Could you check a few things on this model? Use its own coordinates, in mm. Round coordinates to 2 decimals unless told otherwise and drop trailing zeros. Order: outer loops, then holes, each group sorted by start corner. A loop starts at its lowest first (then second) coordinate and runs counter-clockwise, first axis right, second up. Notation, with made-up numbers: (-12.5, 74) -> (46.5, 74) arc R18 cw to (46.5, 92) -> close; hole circle Ø7 at (-34.75, 1). An arc over 180 degrees is marked (long way). One line per question, with ' | ' between items.
```python
from build123d import *

# Parameters (mm, degrees)
F0_W     = 16.9926
F0_H     = 23.0124
F1_DEPTH = 3.175


with BuildPart() as f1:
    # F0 (on Top) → F1 (new body)
    with BuildSketch(Plane.XY):
        Polygon((-38.1, 64.095948), (-38.1, 58.695937), (-38.1, 51.395948), (0, 51.395948), (0, 24.957037), (16.9926, 24.957037), (16.9926, 1.944637), (0, 1.944637), (0, -46.394052), (-38.1, -46.394052), (-38.1, -73.704052), (-38.1, -101.004052), (12.7, -101.004052), (12.7, -126.404052), (-38.1, -126.404052), (-38.1, -139.104052), (127, -139.104052), (127, -126.404052), (76.2, -126.404052), (76.2, -101.004052), (127, -101.004052), (127, -73.704052), (127, -46.394052), (88.9, -46.394052), (88.9, 1.944637), (71.9074, 1.944637), (71.9074, 24.957037), (88.9, 24.957037), (88.9, 51.395948), (127, 51.395948), (127, 58.695937), (127, 64.095948), align=None)
        with Locations((80.4037, 13.450837)):
            Rectangle(F0_W, F0_H)
        with Locations((8.4963, 13.450837)):
            Rectangle(F0_W, F0_H)
        Polygon((12.7, -101.004052), (-38.1, -101.004052), (-38.1, -113.704052), (-38.1, -126.404052), (12.7, -126.404052), align=None)
        Polygon((127, -113.704052), (127, -101.004052), (76.2, -101.004052), (76.2, -126.404052), (127, -126.404052), align=None)
    extrude(amount=F1_DEPTH)


solid = f1.part
```
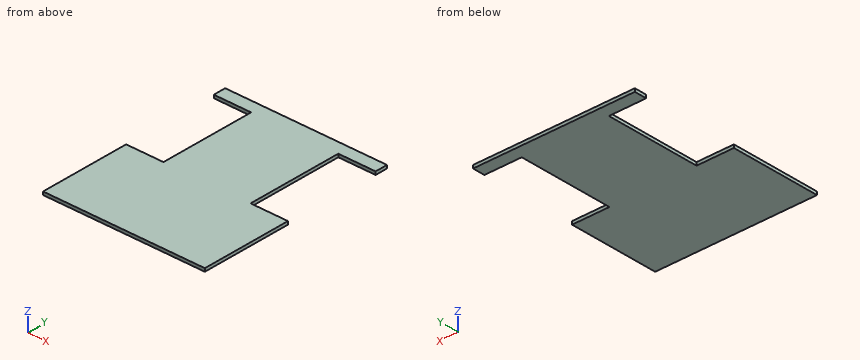
1. I want a section at A-A on x = -24.5. List the corners of the cut face in (y, z) for me (3 decimals).
From the geometry:
outline: (-139.104, 0) -> (-46.394, 0) -> (-46.394, 3.175) -> (-139.104, 3.175) -> close; (51.396, 0) -> (64.096, 0) -> (64.096, 3.175) -> (51.396, 3.175) -> close
2. I'm going to push a flat-ended pin straight in: pin 1 (1 mm diameter, centred on y = 14, z = 2, fed in from -X). Where does the tip first touch, or does it pass through?
From the geometry:
pin 1: stops at x = 0
3. I need wall thicknesses on probe 1 along Y at (x, z) = (-7.5, 0.5); probe 2 along X at (y, z) = (-42.5, 1.1). Which ranges of each line are inside material? Lowest first, please.
From the geometry:
probe 1: y = -139.1 to -46.39, 51.4 to 64.1 | probe 2: x = 0 to 88.9
4. I want a section at C-C on y = 11. List the corners of the cut face in (x, z) for me (3 decimals).
From the geometry:
outline: (0, 0) -> (88.9, 0) -> (88.9, 3.175) -> (0, 3.175) -> close
5. I want a section at B-B on z = 2.45. List the corners of the cut face in (x, y) for me.
From the geometry:
outline: (-38.1, -139.1) -> (127, -139.1) -> (127, -46.39) -> (88.9, -46.39) -> (88.9, 51.4) -> (127, 51.4) -> (127, 64.1) -> (-38.1, 64.1) -> (-38.1, 51.4) -> (0, 51.4) -> (0, -46.39) -> (-38.1, -46.39) -> close
